Input: dimensioned drawing with shaded views. Units: mm. Origin: part minimum x, y, z. Round coordinates to 2 decimals unless told otherwise and drop trailing zeros. Order: outer loops, then holes, each group sorted by start corner. A loop starts at its lowest first (then second) coordinate and runs counter-clockwise, first axis right, second up. Notation, with made-up numbers: M -26.5,-3 L -22.5,-3 A28 ccw -22.5,21 Z; hole C 45.5,57.25 d6. An arc over 180 degrees is marked long. Put each result on its own line as item: value. Start each with the question number.
1) Section A-A, the plane y = 88. Return loops of the section in (x, z), then the cut area to 3 significant figures.
2) Material intervals for probe 1 along Y at (x, z) = (0.65, 17); probe 2 along Y at (x, z) = (1.75, 33.5); probe 3 along Z at (x, y) = (0.2, 42.5), sorted ascending. Write a range as [from, to].
3) Section B-B, the plane z = 108.5. Return loops of the section in (x, y).
4) First-contact query: P1, Ø0.9, axis at x = 2, z = 93, coming from the +Y side; P2, Ø1.5, axis at x = 1.5, y = 94, coming from the -Z side. Flat tips, straight axial feed; report the tip coordinate or a pass-through.
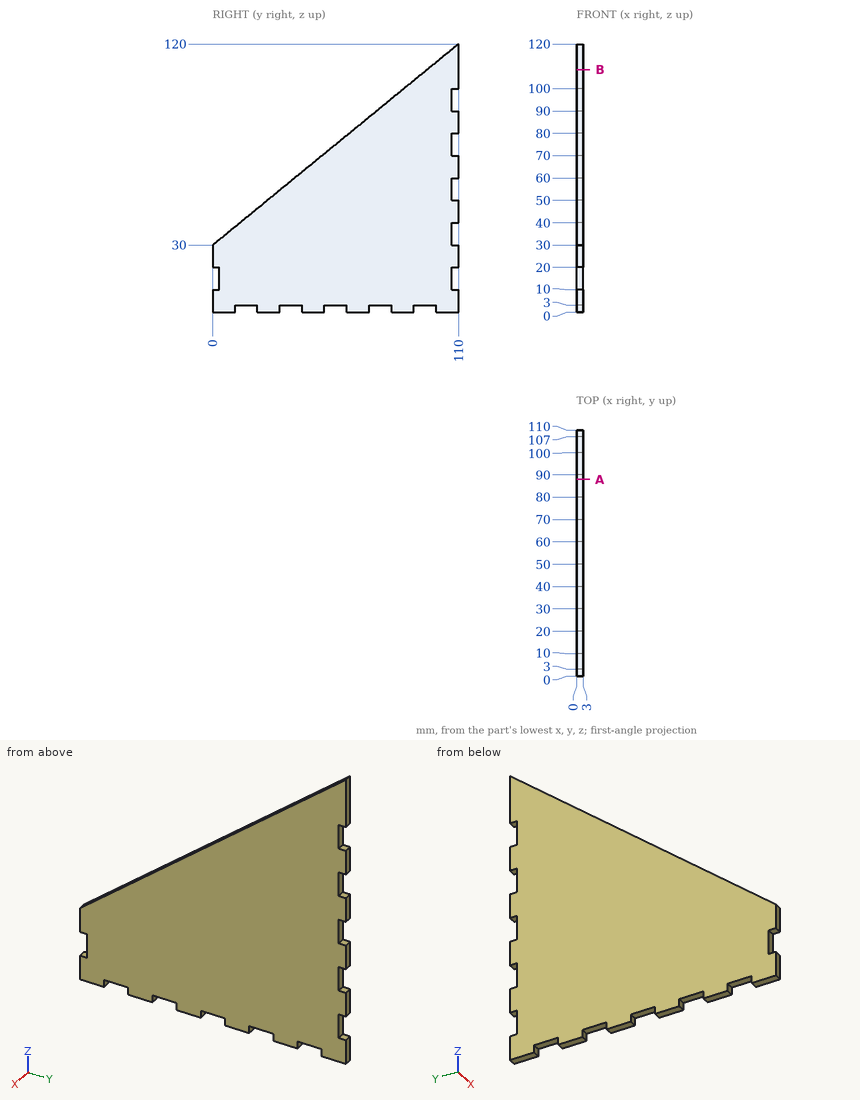
Result sheet:
1. outline: M 0,0 L 3,0 L 3,102 L 0,102 Z
1. area: 306 mm2
2. probe 1: y = [3, 107]
2. probe 2: y = [4.28, 107]
2. probe 3: z = [0, 64.77]
3. outline: M 0,95.94 L 3,95.94 L 3,110 L 0,110 Z
4. P1: stops at y = 107
4. P2: stops at z = 3
